Source: CAD feature listing. Evaluate the final solid. Frame: model axes, mm. Coordinates: 2 decimals unless noted, no trailing zeros.
Item 1: Pin query (flat end, axial travel): pin 1 Ø1 at (x, y) = (1, -0.5) entering from -Z; pin 2 Ø2 at (x, y) = (2.5, -5) entering from -Z; pin 3 Ø1.5 at (x, y) = (0.5, 0) entering from +Z. Return the tip coordinate at first contact, or that it passes through.
Item 2: Section query A-A, the plane y = 3. State how many separate pieces and enclosed holes the cut face has, then the cut area to 3 significant figures.
Item 3: Line query: probe 1 along Y at (x, z) = (2.1, 0.75); probe 2 along Z at (x, y) = (0.5, 4.5); probe 3 along Z at (x, y) = (2.5, -4.25). Output: solid intervals per line, ascending.
```python
from build123d import *

# Parameters (mm, degrees)
BASPROSKE_W     = 3.175
BASPROSKE_H     = 6.985
TOOTHCUT_DEPTH  = 11.375985495
TEETHCUTS_COUNT = 9
BORSKE_R        = 1.5875
BORE_DEPTH      = 50.8000508
SCALE1_SCALE_X  = 1.11
SCALE1_SCALE_Y  = 1
SCALE1_SCALE_Z  = 1.11


with BuildPart() as part:
    # BasProSke → Base-Revolve (revolve)
    with BuildSketch(Plane(origin=(0, 0, 0), x_dir=(1, 0, 0), z_dir=(0, 1, 0)), mode=Mode.PRIVATE) as base_revolve_sk:
        with Locations((1.5875, 3.4925)):
            Rectangle(BASPROSKE_W, BASPROSKE_H)
    revolve(base_revolve_sk.sketch.rotate(Axis((-10, 0, 0), (1, 0, 0)), 180), axis=Axis((-10, 0, 0), (1, 0, 0)))

    # TooCutSke → ToothCut (cut, through all)
    with BuildSketch(Plane(origin=(0, 0, 0), x_dir=(0, 0, -1), z_dir=(1, 0, 0))):
        with BuildLine():
            ThreePointArc((0.85090004, 4.051817513), (0, 4.1402), (-0.85090004, 4.051817513))
            ThreePointArc((-0.85090004, 4.051817513), (-1.187930048, 5.606894235), (-2.458065659, 6.565334826))
            ThreePointArc((-2.458065659, 6.565334826), (0, 7.0104), (2.458065659, 6.565334826))
            ThreePointArc((2.458065659, 6.565334826), (1.187930048, 5.606894235), (0.85090004, 4.051817513))
        make_face()
    toothcut = extrude(amount=TOOTHCUT_DEPTH, mode=Mode.SUBTRACT)

    # TeethCuts: ToothCut ×9 about axis
    teethcuts_axis = Axis((-10, 0, 0), (1, 0, 0))
    for i in range(1, TEETHCUTS_COUNT):
        add(toothcut.rotate(teethcuts_axis, i * 360 / TEETHCUTS_COUNT), mode=Mode.SUBTRACT)

    # BorSke → Bore (cut, symmetric)
    with BuildSketch(Plane(origin=(0, 0, 0), x_dir=(0, 0, -1), z_dir=(1, 0, 0))):
        with Locations(Location((0, 0, 0), (0, 0, 180))):
            Circle(BORSKE_R)
    extrude(amount=BORE_DEPTH, both=True, mode=Mode.SUBTRACT)


with BuildPart() as part_1:
    # Scale1: scaled about (1.5875, 0, 0)
    add(part.part.scale((SCALE1_SCALE_X, SCALE1_SCALE_Y, SCALE1_SCALE_Z), about=(1.5875, 0, 0)))


solid = part_1.part
```
Verdict:
1. pin 1: stops at z = -7.47
1. pin 2: stops at z = -5.02
1. pin 3: stops at z = 7.24
2. separate pieces: 3
2. enclosed holes: 0
2. area: 40.2 mm2
3. probe 1: y = -6.07 to -4.29, -4.08 to -1.44, 1.44 to 4.08
3. probe 2: z = -2.83 to -0.92, 0.92 to 2.83
3. probe 3: z = -4.92 to -2.75, -0.73 to 0.73, 2.75 to 4.92
